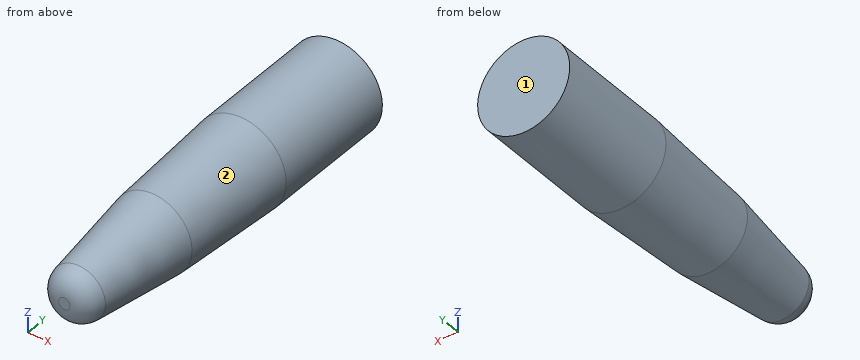
from build123d import *

# Parameters (mm, degrees)
SKETCH_620_R    = 8
EXTRUDE_1_DEPTH = 23


# Read off the part's stored shape, not the designer's step: 凸台-拉伸2
with BuildPart() as part:
    # Sketch 620 → 凸台-拉伸1 (new body)
    with BuildSketch(Plane(origin=(0, 0, 0), x_dir=(1, 0, 0), z_dir=(0, 1, 0))):
        with Locations(Location((0, 0, 0), (0, 0, 270))):
            Circle(SKETCH_620_R)
    extrude(amount=EXTRUDE_1_DEPTH)

    # 凸台-拉伸2 outline → 凸台-拉伸2 (revolve)
    with BuildSketch(Plane.XY):
        Polygon((0, -21), (6.899436635, -21), (8, 0), (0, 0), align=None)
    revolve(axis=Axis((0, 0, 0), (0, 1, 0)))

    # 草图7 → 旋转4 (revolve)
    with BuildSketch(Plane.XY, mode=Mode.PRIVATE) as revolve_4_sk:
        with BuildLine():
            Line((0, -21), (6.899436635, -21))
            Line((6.899436635, -21), (4.725684175, -38.703793083))
            ThreePointArc((4.725684175, -38.703793083), (3.487252632, -41.057664274), (1, -42))
            Line((1, -42), (0, -42))
            Line((0, -42), (0, -21))
        make_face()
    revolve(revolve_4_sk.sketch.rotate(Axis((0, -21, 0), (0, -1, 0)), 180), axis=Axis((0, -21, 0), (0, -1, 0)))


solid = part.part
Check sheet for the modelled part. Datum: model origin and axes. Units: mm. Face numbers are marked on the shaded views. Round coordinates to 2 decimals unless told otherwise and drop trailing zeros. Loops run counter-clockwise (first coordinate to the right, second up) from the corner with the lowest first, then second, coordinate; pieces in that order, holes last. Notation, with made-up numbers: (28.5, -21.75) -> (53.5, -21.75) arc R19 cw to (53.5, -13.75) -> close; hole circle Ø6 at (57, 3.25). An arc over 180 degrees is marked (long way). Put each result on its own line as item: value. Start each with the question number.
1. Section check A-A (y = 15). Enter the section's corners in (x, z), plus the area to 3 significant figures.
2. Draft check along X on the marked faces 1 and 2. Enter one of: +X half, -X half, draft (parallel to the pull), parting line (faces both ways), or undercut.
3. Gauge pin test, flat ends, axial feed: pin 1 (3 mm diameter, centred on y = -25.5, z = 2.5, fed in from +X); pin 2 (1.5 mm diameter, centred on x = 1.5, y = 2.5, fed in from +Z); pin 3 (5 mm diameter, centred on x = 2, y = 7, fed in from -Z); pin 4 (1.5 mm diameter, centred on x = 4.5, z = 0.5, fed in from -Y). Record the tip position at first contact, or that the pin passes through.
4. Scan lines: probe 1 along Z at (x, y) = (-7, -1.5); probe 2 along Z at (x, y) = (4.25, -29.5); probe 3 along X at (y, z) = (-27, 0.75). Record each from-to range of solid material in increasing order.
Findings:
1. outline: circle Ø16 at (0, 0)
1. area: 201 mm^2
2. face 1: draft
2. face 2: parting line
3. pin 1: stops at x = 6.33
3. pin 2: stops at z = 7.96
3. pin 3: stops at z = -8
3. pin 4: stops at y = -40.77
4. probe 1: z = -3.71 to 3.71
4. probe 2: z = -4.03 to 4.03
4. probe 3: x = -6.12 to 6.12
